```python
from build123d import *

# Parameters (mm, degrees)
F0_R     = 2.347977
F0_R_2   = 3.175
F0_R_3   = 1.5875
F1_DEPTH = 3.175


with BuildPart() as f1:
    # F0 (on Front) → F1 (new body)
    with BuildSketch(Plane.XZ):
        with BuildLine():
            Line((-85.725, -25.4), (-10.55478, -12.517509))
            ThreePointArc((-10.55478, -12.517509), (-2.990873, -8.186748), (0, 0))
            Line((0, 0), (-84.1375, 0))
            ThreePointArc((-84.1375, 0), (-86.506722, -1.38169), (-86.542623, 1.360753))
            Line((-86.542623, 1.360753), (-98.806967, 21.772049))
            ThreePointArc((-98.806967, 21.772049), (-110.201214, -6.787855), (-85.725, -25.4))
        make_face()
        with Locations((-92.075, -9.525)):
            Circle(F0_R, mode=Mode.SUBTRACT)
        with Locations((-101.6, -3.175)):
            Circle(F0_R_2, mode=Mode.SUBTRACT)
        with Locations((-76.2, -12.7)):
            Circle(F0_R_3, mode=Mode.SUBTRACT)
        with Locations((-47.625, -9.525)):
            Circle(F0_R_3, mode=Mode.SUBTRACT)
        with Locations((-19.05, -6.35)):
            Circle(F0_R_3, mode=Mode.SUBTRACT)
    extrude(amount=F1_DEPTH)


solid = f1.part
```
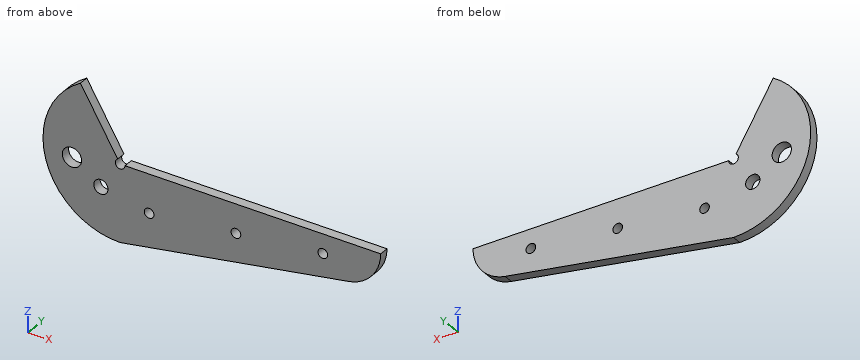
Source: CAD feature listing. Evaluate the final solid. Frame: model axes, mm. Give positions to 0.01 mm unless a question says otherwise; leave off trailing zeros. Write each loop counter-clockwise with the first axis right and the second up, starting at its lowest first coordinate (ties: lowest second). Pieces come first, ordered by that corner, then holes.
1. First-contact query: pin 1 (2.5 mm diameter, centred on x = -47.625, z = -9.525, fed in from -Y); pin 2 (1.5 mm diameter, centred on y = -1, z = 8.5, fed in from -X); pin 3 (1.5 mm diameter, centred on x = -25, y = -1.5, fed in from +Z); pin 4 (10 mm diameter, centred on x = -35.5, z = -20, fed in from +Y). Flat tips, straight axial feed; report the tip coordinate or a pass-through.
2. Section query B-B (y = -1.9). Count the separate pieces of the cut face and the enclosed holes in it, then the cut area to 3 significant figures.
3. Section query D-D (x = -76.2). Return the cut outline in (y, z) (1 decimal).
4. Material intervals for line 1 along X through (y, z) = (-2.1, -8.5); line 2 along Z through (x, y) = (-19.05, -0.9); line 3 along X through (y, z) = (-1.7, -7.5), sorted ascending.
5. Section query A-A (x = -19.05). Return the cut outline in (y, z) (1 decimal).
6. Section query C-C (z = 16.5). Return the cut outline in (x, y) (3 decimals), then the cut area to 3 significant figures.
Output values:
1. pin 1: passes through
1. pin 2: stops at x = -109.91
1. pin 3: stops at z = 0
1. pin 4: stops at y = 0
2. separate pieces: 1
2. enclosed holes: 5
2. area: 2,290 mm2
3. outline: (-3.2, -23.8) - (0, -23.8) - (0, -14.3) - (-3.2, -14.3) - close; (-3.2, -11.1) - (0, -11.1) - (0, 0) - (-3.2, 0) - close
4. line 1: x = -109.66 to -94.19, -89.96 to -48.84, -46.41 to -3.26
4. line 2: z = -13.97 to -7.94, -4.76 to 0
4. line 3: x = -109.99 to -93.26, -90.89 to -20.14, -17.96 to -2.45
5. outline: (-3.2, -14) - (0, -14) - (0, -7.9) - (-3.2, -7.9) - close; (-3.2, -4.8) - (0, -4.8) - (0, 0) - (-3.2, 0) - close
6. outline: (-105.036, -3.175) - (-95.639, -3.175) - (-95.639, 0) - (-105.036, 0) - close
6. area: 29.8 mm2
